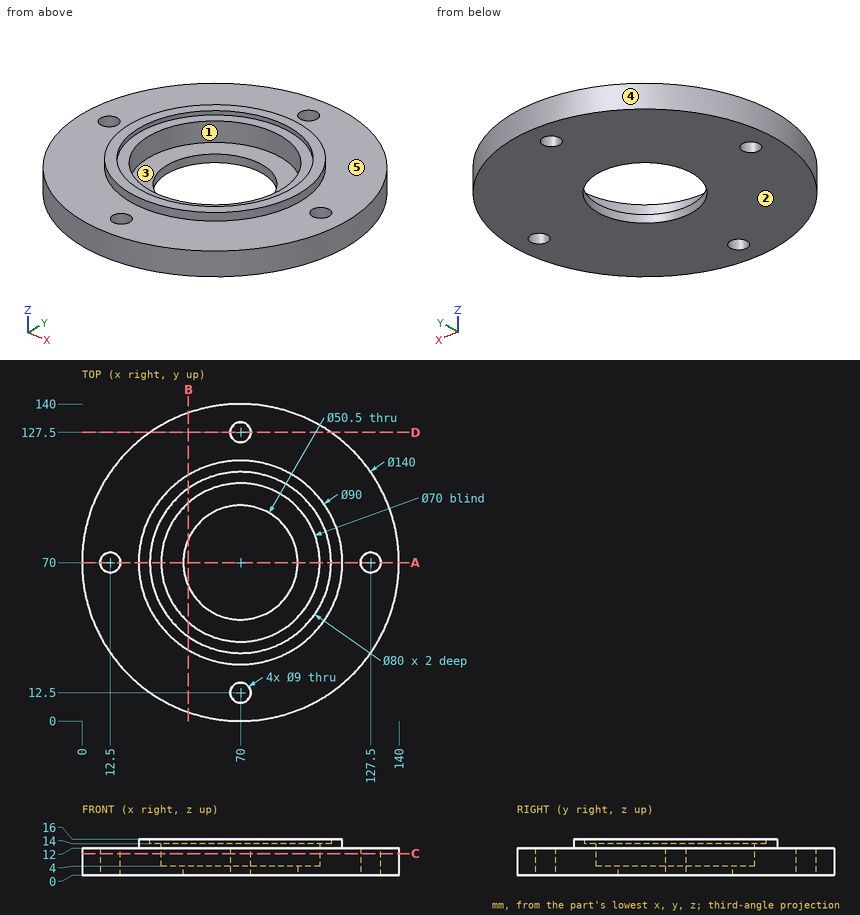
Geometry check sheet. Reference: drawing and pictorial views, mm from the part's lowest x, y, z. A direction names the side the tool comes from. Give positions to 0.01 mm unless a question says otherwise; leave off trailing zeros. Write each loop counter-clockwise with the first axis right and the second up, starting at its lowest first coordinate (ties: lowest second). Pieces come first, ordered by that corner, then holes. Notation, with made-up numbers: (24, 48.5) - (38, 48.5) arc R13 ccw to (38, 57.5) - close; hole circle Ø10 at (-36, -3). An arc over 180 degrees is marked (long way). Use a Markdown table: item, result.
Q1. Section check C-C, the plane z = 9.5. Enter the section's corners in (x, y).
Computed:
| item | result |
|---|---|
| outline | circle Ø140 at (70, 70); hole circle Ø9 at (12.5, 70); hole circle Ø70 at (70, 70); hole circle Ø9 at (70, 12.5); hole circle Ø9 at (70, 127.5); hole circle Ø9 at (127.5, 70) |
Q2. Draft check along Y on the marked faces 3, 4 and 5. Enter one of: pulls with the +Y half, pulls with the -Y half, needs draft (parallel to the pull), parting line crosses it, or undercut.
Computed:
| item | result |
|---|---|
| face 3 | undercut |
| face 4 | parting line crosses it |
| face 5 | needs draft |
Q3. Go/stop test with flat-tipped pins: P1, Ø14.5, axis at x = 127.5, y = 70, coming from the +Z side; P2, Ø4, axis at x = 77, z = 8.5, coming from the +Y side; P3, Ø1, axis at y = 37.5, z = 4, coming from the +X side. Record where each tip stops, or that it passes through.
Computed:
| item | result |
|---|---|
| P1 | stops at z = 12 |
| P2 | stops at y = 139.82 |
| P3 | stops at x = 132.26 |
Q4. Set-up check for the marked faces 1 and 2: record each of +Z, -Z, +X, -X, +Y, -Y from which the full face is reachable in a straight line by a thin tool's end or side.
Computed:
| item | result |
|---|---|
| face 1 | +Z |
| face 2 | -Z, +X, -X, +Y, -Y |
Q5. Section check B-B, the plane x = 47. Enter the section's corners in (y, z), then the cut area to 3 significant figures.
Computed:
| item | result |
|---|---|
| outline | (3.89, 0) - (59.58, 0) - (59.58, 4) - (43.62, 4) - (43.62, 14) - (37.27, 14) - (37.27, 16) - (31.32, 16) - (31.32, 12) - (3.89, 12) - close; (80.42, 0) - (136.11, 0) - (136.11, 12) - (108.68, 12) - (108.68, 16) - (102.73, 16) - (102.73, 14) - (96.38, 14) - (96.38, 4) - (80.42, 4) - close |
| area | 1,150 mm² |
Q6. Section check A-A, the plane y = 70. Enter the section's corners in (x, z), then the cut area to 3 significant figures.
Computed:
| item | result |
|---|---|
| outline | (0, 0) - (8, 0) - (8, 12) - (0, 12) - close; (17, 0) - (44.75, 0) - (44.75, 4) - (35, 4) - (35, 14) - (30, 14) - (30, 16) - (25, 16) - (25, 12) - (17, 12) - close; (95.25, 0) - (123, 0) - (123, 12) - (115, 12) - (115, 16) - (110, 16) - (110, 14) - (105, 14) - (105, 4) - (95.25, 4) - close; (132, 0) - (140, 0) - (140, 12) - (132, 12) - close |
| area | 762 mm² |
Q7. Section check D-D, the plane y = 127.5. Enter the section's corners in (x, z).
Computed:
| item | result |
|---|---|
| outline | (30.08, 0) - (65.5, 0) - (65.5, 12) - (30.08, 12) - close; (74.5, 0) - (109.92, 0) - (109.92, 12) - (74.5, 12) - close |
Q8. Thickness scan on L1, parallel to Y at x = 70, z = 8.5; L2, parallel to Z at x = 99, y = 28; L3, parallel to Y at x = 127, z = 10.5. Record the ranges inside material, lowest first. Write a range as [from, to].
Computed:
| item | result |
|---|---|
| L1 | y = [0, 8], [17, 35], [105, 123], [132, 140] |
| L2 | z = [0, 12] |
| L3 | y = [29.37, 65.53], [74.47, 110.63] |
